```python
from build123d import *

# Parameters (mm, degrees)
F0_W     = 10
F0_H     = 10
F0_W_2   = 8
F0_H_2   = 8
F1_DEPTH = 61
F2_R     = 1.5
F3_DEPTH = 25
F4_R     = 1.5
F5_DEPTH = 25


with BuildPart() as f1:
    # F0 (on Front) → F1 (new body)
    with BuildSketch(Plane.XZ):
        Rectangle(F0_W, F0_H)
        Rectangle(F0_W_2, F0_H_2, mode=Mode.SUBTRACT)
    extrude(amount=F1_DEPTH)

    # F2 (on face) → F3 (cut)
    with BuildSketch(Plane.XY.offset(5)):
        with Locations((0, -5)):
            Circle(F2_R)
        with Locations((0, -56)):
            Circle(F2_R)
    extrude(amount=-F3_DEPTH, mode=Mode.SUBTRACT)

    # F4 (on face) → F5 (cut)
    with BuildSketch(Plane.YZ.offset(5)):
        with Locations((-15, -1)):
            Circle(F4_R)
        with Locations((-46, -1)):
            Circle(F4_R)
    extrude(amount=-F5_DEPTH, mode=Mode.SUBTRACT)


solid = f1.part
```
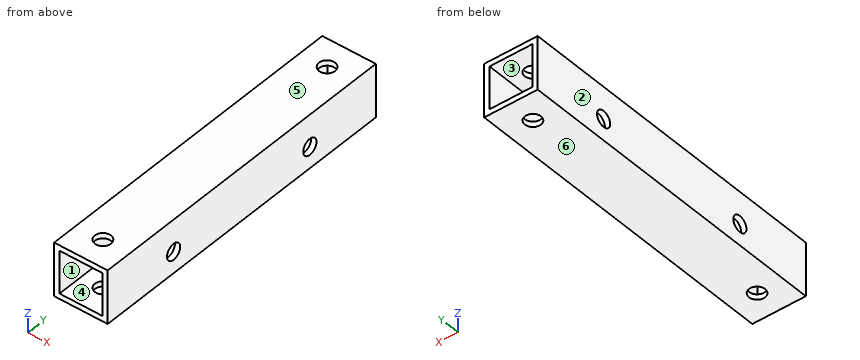
Build history of the part. All positions in model axes, mm. Face numbers are marked on the shaded views. A direction names the side the tool comes from. Round coordinates to 2 decimals unless told otherwise and drop trailing zeros. Write each loop counter-clockwise with the first axis right and the second up, starting at its lowest first coordinate (ties: lowest second). Pieces come first, ordered by that corner, then holes. Notation, with made-up numbers: (52.25, 11.25) - (70.25, 11.25) arc R12 ccw to (70.25, 32.25) - close; hole circle Ø9 at (58, 24). An arc over 180 degrees is marked (long way). Write each question's results on one line, items separated by ' | '. Start each with the question number.
Item 1: Which spindle directions (+Z, -Z, +X, -X, +Y, -Y) get a long thin tool onto all of the face, cutting with end or side? Do the marked faces 1 and 2. Say none if no direction does.
Item 2: Mould opens along Z. For the marked faces 3, 4, 5 and 6 say: pulls with the +Z half, pulls with the -Z half, needs draft (parallel to the pull), parting line crosses it, or undercut.
Item 3: Saw through at D-D (x = 0). Write the cut outline in (y, z), and give its area (3 significant figures).
Item 4: Saw through at B-B (x = -2.75). Write the cut outline in (y, z), and give its area (3 significant figures).
Item 5: Wall check: L1, parallel to Y at x = 0, z = -4.55; L2, parallel to X at y = -30.5, z = -2.75. Give the ranges that are in metal, low to high. Write a range as [from, to].
Item 6: Saw through at A-A (z = -1). Write the cut outline in (x, y).
Item 7: Saw through at C-C (y = -5). Write the cut outline in (x, z), and give its area (3 significant figures).
Results are:
1) face 1: +Y, -Y | face 2: +Z, -Z, -X, +Y, -Y
2) face 3: undercut | face 4: undercut | face 5: pulls with the +Z half | face 6: pulls with the -Z half
3) outline: (-61, -5) - (-57.5, -5) - (-57.5, -4) - (-61, -4) - close; (-61, 4) - (-57.5, 4) - (-57.5, 5) - (-61, 5) - close; (-54.5, -5) - (-6.5, -5) - (-6.5, -4) - (-54.5, -4) - close; (-54.5, 4) - (-6.5, 4) - (-6.5, 5) - (-54.5, 5) - close; (-3.5, -5) - (0, -5) - (0, -4) - (-3.5, -4) - close; (-3.5, 4) - (0, 4) - (0, 5) - (-3.5, 5) - close | area: 110 mm²
4) outline: (-61, -5) - (0, -5) - (0, -4) - (-61, -4) - close; (-61, 4) - (0, 4) - (0, 5) - (-61, 5) - close | area: 122 mm²
5) L1: y = [-61, -57.5], [-54.5, -6.5], [-3.5, 0] | L2: x = [-5, -4], [4, 5]
6) outline: (-5, -61) - (-4, -61) - (-4, -47.5) - (-5, -47.5) - close; (-5, -44.5) - (-4, -44.5) - (-4, -16.5) - (-5, -16.5) - close; (-5, -13.5) - (-4, -13.5) - (-4, 0) - (-5, 0) - close; (4, -61) - (5, -61) - (5, -47.5) - (4, -47.5) - close; (4, -44.5) - (5, -44.5) - (5, -16.5) - (4, -16.5) - close; (4, -13.5) - (5, -13.5) - (5, 0) - (4, 0) - close
7) outline: (-5, -5) - (-1.5, -5) - (-1.5, -4) - (-4, -4) - (-4, 4) - (-1.5, 4) - (-1.5, 5) - (-5, 5) - close; (1.5, -5) - (5, -5) - (5, 5) - (1.5, 5) - (1.5, 4) - (4, 4) - (4, -4) - (1.5, -4) - close | area: 30.0 mm²
